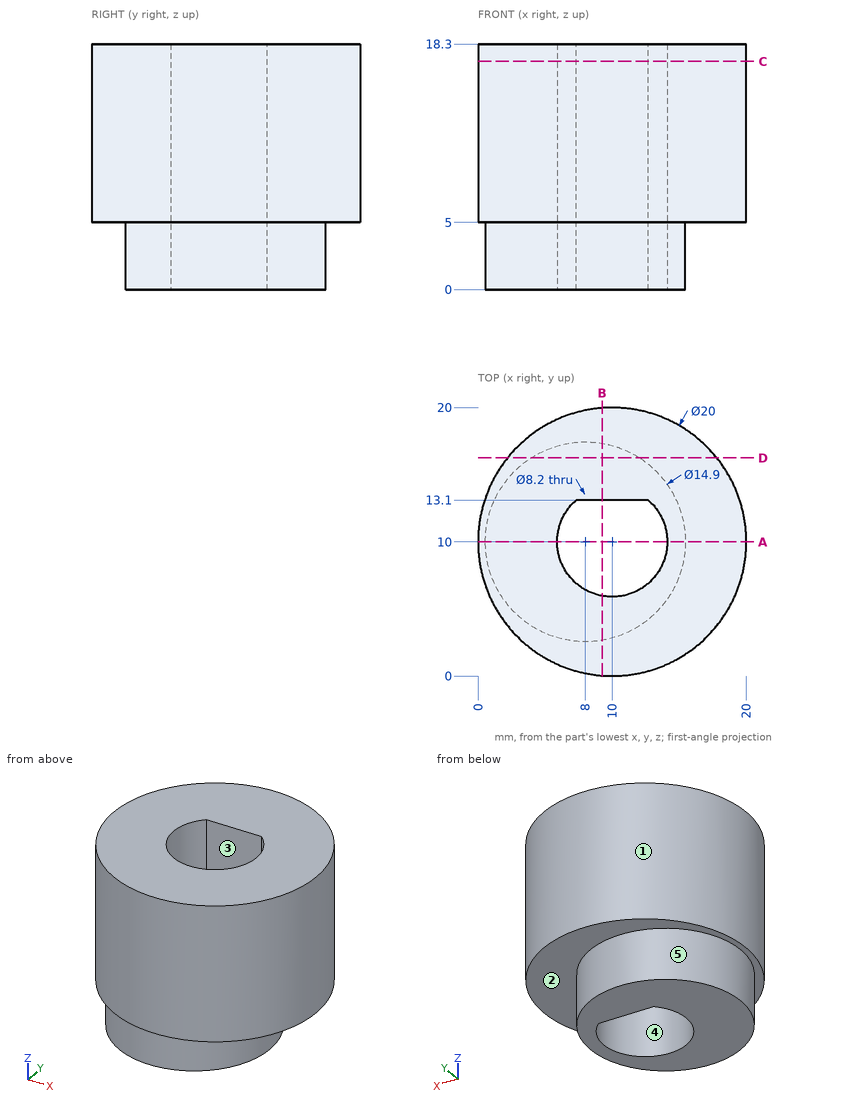
Design review of the part shown in the three views and the two pictorial views. Dimensions are in mm from the part's minimum x, y and z. A direction names the side the tool comes from. Round coordinates to 2 decimals unless told otherwise and drop trailing zeros. Loops run counter-clockwise (first coordinate to the right, second up) from the corner with the lowest first, then second, coordinate; pieces in that order, holes last.
Q1. Add section C-C on z = 17. Write out the cut boundary in (x, y).
Result sheet:
outline: circle Ø20 at (10, 10); hole (7.32, 13.1) arc R4.1 ccw (long way) to (12.68, 13.1) - close
Q2. Insertion check: pin 1 Ø4 at (x, z) = (3.5, 4.5) entering from +Y; pin 2 Ø5 at (x, z) = (16, 5) entering from -Y; pin 3 Ø8 at (y, z) = (16, 11) entering from +X. Each pin has a flat end and moves straight along its axis. Give the tip position at first contact, or say it passes through.
Result sheet:
pin 1: stops at y = 18.9
pin 2: stops at y = 0.63
pin 3: stops at x = 19.8
Q3. Add section B-B on x = 9.25. Write out the cut boundary in (y, z).
Result sheet:
outline: (0.03, 5) - (2.66, 5) - (2.66, 0) - (5.97, 0) - (5.97, 18.3) - (0.03, 18.3) - close; (13.1, 0) - (17.34, 0) - (17.34, 5) - (19.97, 5) - (19.97, 18.3) - (13.1, 18.3) - close
Q4. Mouldability with a two-part tool opening along Y and no side actions: class the marked faces 1, 2 and 3 as +Y half, -Y half, draft (parallel to the pull), parting line (faces both ways), or undercut.
Result sheet:
face 1: parting line
face 2: draft
face 3: undercut
Q5. Machinability: for the marked faces 4 and 5, which of the approach directions +Z, -Z, +X, -X, +Y, -Y give a long, thin tool a straight path to every point of the face, cutting with its end or side? Answer none if there is none.
Result sheet:
face 4: +Z, -Z
face 5: -Z
Q6. To check wall thickness, follow line 1 along Y through (x, z) = (10, 6.75); line 2 along Y through (x, z) = (13.25, 5.75); line 3 along Z through (x, y) = (1.25, 5.25). State the ranges of each line that lie inside material, in increasing order.
Result sheet:
line 1: y = 0 to 5.9, 13.1 to 20
line 2: y = 0.54 to 7.5, 12.5 to 19.46
line 3: z = 5 to 18.3
Q7. Add section A-A on y = 10. Write out the cut boundary in (x, z).
Result sheet:
outline: (0, 5) - (0.55, 5) - (0.55, 0) - (5.9, 0) - (5.9, 18.3) - (0, 18.3) - close; (14.1, 0) - (15.45, 0) - (15.45, 5) - (20, 5) - (20, 18.3) - (14.1, 18.3) - close
Q8. Add section D-D on y = 16.25. Write out the cut boundary in (x, z).
Result sheet:
outline: (2.19, 5) - (3.95, 5) - (3.95, 0) - (12.05, 0) - (12.05, 5) - (17.81, 5) - (17.81, 18.3) - (2.19, 18.3) - close
